```python
from build123d import *

# Parameters (mm, degrees)
F1_DEPTH = 450
F2_R     = 5
F3_R     = 7
F4_R     = 2.6
F5_DEPTH = 25


with BuildPart() as f1:
    # F0 (on Front) → F1 (new body)
    with BuildSketch(Plane.XZ):
        Polygon((-67.5, 2), (-67.5, 0), (-44.5, 0), (-44.5, -63), (0, -63), (44.5, -63), (44.5, 0), (67.5, 0), (67.5, 2), (42.5, 2), (42.5, -61), (0, -61), (-42.5, -61), (-42.5, 2), align=None)
    extrude(amount=F1_DEPTH)

    # F2
    f2_edges = [f1.edges().sort_by_distance(p)[0] for p in [
        (-42.5, -225, -61),
        (44.5, -225, 0),
        (-44.5, -225, 0),
        (42.5, -225, -61),
    ]]
    fillet(f2_edges, radius=F2_R)

    # F3
    f3_edges = [f1.edges().sort_by_distance(p)[0] for p in [
        (-42.5, -225, 2),
        (44.5, -225, -63),
        (42.5, -225, 2),
        (-44.5, -225, -63),
    ]]
    fillet(f3_edges, radius=F3_R)

    # F4 (on face) → F5 (cut)
    with BuildSketch(Plane.XY.offset(2)):
        with Locations((58.5, -425)):
            Circle(F4_R)
        with Locations((58.5, -325)):
            Circle(F4_R)
        with Locations((58.5, -125)):
            Circle(F4_R)
        with Locations((58.5, -25)):
            Circle(F4_R)
        with Locations((-58.5, -25)):
            Circle(F4_R)
        with Locations((-58.5, -125)):
            Circle(F4_R)
        with Locations((-58.5, -325)):
            Circle(F4_R)
        with Locations((-58.5, -425)):
            Circle(F4_R)
    extrude(amount=-F5_DEPTH, mode=Mode.SUBTRACT)


solid = f1.part
```
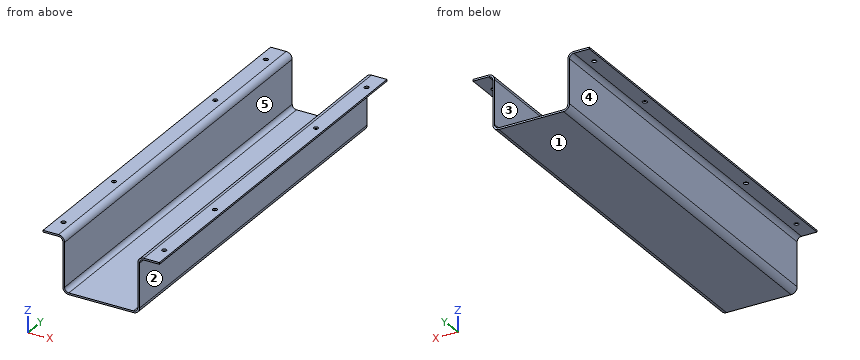
Geometry: final body of the model. Coordinates: model frame, mm. Face numbers are marked on the shaded views. A direction names the side the tool comes from. Round coordinates to 2 decimals unless told otherwise and drop trailing zeros. Loops run counter-clockwise (first coordinate to the right, second up) from the corner with the lowest first, then second, coordinate; pieces in that order, holes last. Notation, with made-up numbers: (59.5, -20) -> (87.5, -20) arc R27 ccw to (87.5, 6) -> close; hole circle Ø9 at (31, -30.75). An arc over 180 degrees is marked (long way). Write each question's results on one line, items separated by ' | '.
Item 1: Pull-direction query (X, two-part tool) for the marked faces 1, 2 and 3; classes: pulls with the +X half, pulls with the -X half, needs draft (parallel to the pull), parting line crosses it, or undercut.
Answers below:
face 1: needs draft | face 2: pulls with the +X half | face 3: undercut
Item 2: Pin query (flat end, axial travel): pin 1 Ø4 at (y, z) = (-166, -36.5) entering from -X; pin 2 Ø9 at (x, y) = (55, -312) entering from -Z; pin 3 Ø6 at (x, y) = (-34.5, -205.5) entering from +Z; pin 4 Ø4 at (x, z) = (39, -22.5) entering from -Y. Return the tip coordinate at first contact, or that it passes through.
Answers below:
pin 1: stops at x = -44.5 | pin 2: stops at z = 0 | pin 3: stops at z = -61 | pin 4: passes through
Item 3: Cut plane B-B on x = 23. Return the cut outline in (y, z), and give its area (3 significant figures).
Answers below:
outline: (-450, -63) -> (0, -63) -> (0, -61) -> (-450, -61) -> close | area: 900 mm²
Item 4: Set-up query: the marked faces 4 and 5. Return all of +Z, -Z, +X, -X, +Y, -Y with unobstructed straight access to the full face (end or side cutting, diameter ignored); none if empty.
Answers below:
face 4: -Z, -X, +Y, -Y | face 5: +Z, +Y, -Y
Item 5: Cut plane A-A on z = -39.5. Return the cut outline in (x, y), and give its area (3 significant figures).
Answers below:
outline: (-44.5, -450) -> (-42.5, -450) -> (-42.5, 0) -> (-44.5, 0) -> close; (42.5, -450) -> (44.5, -450) -> (44.5, 0) -> (42.5, 0) -> close | area: 1,800 mm²
Item 6: Line query: probe 1 along Y at (x, z) = (58, 1); probe 2 along X at (y, z) = (-178.5, -51.5); probe 3 along Z at (x, y) = (-36, -385.5). Output: solid intervals per line, ascending. Write a range as [from, to].
Answers below:
probe 1: y = [-450, -427.55], [-422.45, -327.55], [-322.45, -127.55], [-122.45, -27.55], [-22.45, 0] | probe 2: x = [-44.5, -42.5], [42.5, 44.5] | probe 3: z = [-63, -61]
